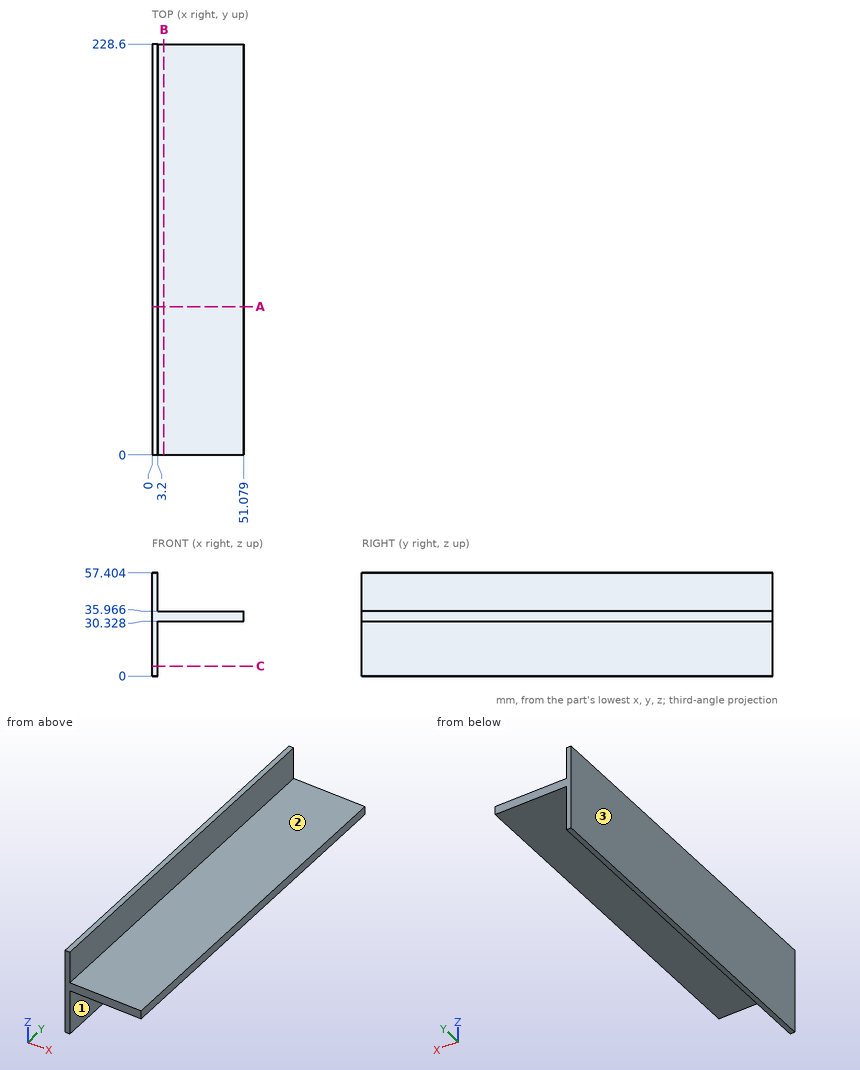
Answer from the drawing. Dimensions are ordinates in mm from the lowest x, y and z of the part. A direction names the side the tool comes from. Round coordinates to 2 decimals unless told otherwise and drop trailing zeros. Loops run counter-clockwise (first coordinate to the right, second up) from the corner with the lowest first, then second, coordinate; pieces in that order, holes last. Notation, with made-up numbers: (4, 60.5) - (17, 60.5) arc R12 cw to (17, 68.5) - close; hole circle Ø3 at (47, -37). An arc over 180 degrees is marked (long way). Return JSON: item names as keys, results as strings. Group by question number.
1. Which of the six approach directions +Z, -Z, +X, -X, +Y, -Y give full straight-line access (tool end or side, diameter ignored) to the marked faces 1, 2 and 3?
2. The part is cut by section A-A on y = 82.5. Determine the outline of the cut face in (x, z).
3. Each of these flat-tipped pins is pushed along its axis until it touches: P1, Ø12, axis at x = 39.5, y = 56, coming from the -Z side; P2, Ø6, axis at x = 44.5, y = 147, coming from the +Z side; P3, Ø8, axis at y = 174, z = 13.5, coming from the +X side. Where does it stop, or does it pass through?
4. The part is cut by section C-C on z = 5.5. Determine the outline of the cut face in (x, y).
5. The part is cut by section B-B on x = 6.5. Determine the outline of the cut face in (y, z), then the cut area to 3 significant figures.
6. Consider probe 1 along Z at (x, y) = (6, 106.5); probe 2 along X at (y, z) = (164.5, 19). Determine where each line is inside the solid, lowest interval first.
Resolved:
{
 "1": {"face 1": "-Z, +X, +Y, -Y", "face 2": "+Z, +X, +Y, -Y", "face 3": "+Z, -Z, -X, +Y, -Y"},
 "2": {"outline": "(0, 0) - (3.2, 0) - (3.2, 30.33) - (51.08, 30.33) - (51.08, 35.97) - (3.2, 35.97) - (3.2, 57.4) - (0, 57.4) - close"},
 "3": {"P1": "stops at z = 30.33", "P2": "stops at z = 35.97", "P3": "stops at x = 3.2"},
 "4": {"outline": "(0, 0) - (3.2, 0) - (3.2, 228.6) - (0, 228.6) - close"},
 "5": {"outline": "(0, 30.33) - (228.6, 30.33) - (228.6, 35.97) - (0, 35.97) - close", "area": "1,290 mm²"},
 "6": {"probe 1": "z = 30.33 to 35.97", "probe 2": "x = 0 to 3.2"}
}
